from build123d import *

# Parameters (mm, degrees)
SKETCH_1_R               = 59
EXTRUDE_1_DEPTH          = 40
FILLET_1_R               = 10
SKETCH_2_R               = 5
EXTRUDE_2_DEPTH          = 5
SKETCH_3_R               = 1.75
EXTRUDE_3_DEPTH          = 5
CUT_EXTRUDE_1_DEPTH      = 93.531075925
PATTERN_CIRCULAR_1_COUNT = 6


with BuildPart() as part:
    # 草图1 → 凸台-拉伸1 (new body)
    with BuildSketch(Plane.XY):
        Circle(SKETCH_1_R)
    extrude(amount=EXTRUDE_1_DEPTH)

    # 圆角1
    fillet_1_edges = [part.edges().sort_by_distance(p)[0] for p in [
        (-59, 0, 0),
        (-59, 0, 40),
    ]]
    fillet(fillet_1_edges, radius=FILLET_1_R)

    # 草图2 → 凸台-拉伸2 (add)
    with BuildSketch(Plane.XY.offset(40)):
        Circle(SKETCH_2_R)
    extrude(amount=EXTRUDE_2_DEPTH)

    # 草图3 → 凸台-拉伸3 (add)
    with BuildSketch(Plane.XY.offset(45)):
        Circle(SKETCH_3_R)
    extrude(amount=EXTRUDE_3_DEPTH)

    # 草图4 → 切除-拉伸1 (cut, through all)
    with BuildSketch(Plane.XY.offset(40)):
        with BuildLine():
            Line((-9.6, 32.2), (-2.88, 9.16))
            ThreePointArc((-2.88, 9.16), (0, 7), (2.88, 9.16))
            Line((2.88, 9.16), (9.6, 32.2))
            ThreePointArc((9.6, 32.2), (0, 45), (-9.6, 32.2))
        make_face()
    cut_extrude_1 = extrude(amount=-CUT_EXTRUDE_1_DEPTH, mode=Mode.SUBTRACT)

    # 阵列(圆周)1: 切除-拉伸1 ×6 about axis
    pattern_circular_1_axis = Axis((0, 0, 0), (0, 0, 1))
    for i in range(1, PATTERN_CIRCULAR_1_COUNT):
        add(cut_extrude_1.rotate(pattern_circular_1_axis, i * 360 / PATTERN_CIRCULAR_1_COUNT), mode=Mode.SUBTRACT)


solid = part.part
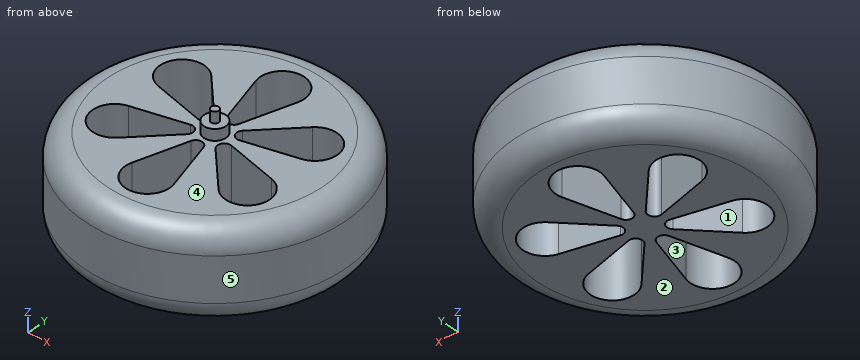
Source: CAD feature listing. Evaluate the final solid. Frame: model axes, mm. Face numbers are marked on the shaded views. A direction names the side the tool comes from. Round coordinates to 2 decimals unless told otherwise and drop trailing zeros. Loops run counter-clockwise (first coordinate to the right, second up) from the corner with the lowest first, then second, coordinate; pieces in that order, holes last. Notation, with made-up numbers: (25.25, -25) - (50.25, -25) arc R18 cw to (50.25, 8) - close; hole circle Ø9 at (-4.5, -36.5). An arc over 180 degrees is marked (long way). Write item = value, one per line. Start each with the question number.
Item 1: First-contact query: pin 1 Ø18 at (x, y) = (0, -35) entering from -Z; pin 2 Ø12 at (x, y) = (42.5, 38.5) entering from -Z; pin 3 Ø6 at (x, y) = (36, 1) entering from +Z; pin 4 Ø2 at (x, z) = (-28.5, 37) entering from -Y. Flat tips, straight axial feed; report the tip coordinate or a pass-through.
Item 2: Mould query, pull axis Y, two halves, no side actions, for the marked faces 3, 4 and 5. Classes: released by +Y, released by -Y, zero draft, split by the parting line, or undercut.
Item 3: Section query B-B on y = 0. Output: boundary loops of the cut face in (x, z), plus the area to 3 significant figures.
Item 4: Reachability of the marked faces 1 and 2 from +Z, -Z, +X, -X, +Y, -Y: full face, straight path, thin tool, end or side. Return the list, or none.
Item 5: Material intervals for line 1 (Y direction, x = 0, z = 29.5); line 2 (Y direction, x = 20, z = 9); line 3 (X direction, y = -19, z = 5), sorted ascending.
Item 6: Section query D-D on x = -12. Count the separate pieces of the cut face and the enclosed holes in it, plus the area to 3 significant figures.
Item 7: Section query C-C on z = 41.5. Output: boundary loops of the cut face in (x, y), plus the area to 3 significant figures.
Item 8: Section query A-A on z = 16. Output: boundary loops of the cut face in (x, y), plus the area to 3 significant figures.
Results list:
q1.pin_1 = through
q1.pin_2 = 0.28
q1.pin_3 = 40
q1.pin_4 = -49.53
q2.face_3 = undercut
q2.face_4 = zero draft
q2.face_5 = split by the parting line
q3.outline = (-59, 10) arc R10 ccw to (-49, 0) - (49, 0) arc R10 ccw to (59, 10) - (59, 30) arc R10 ccw to (49, 40) - (5, 40) - (5, 45) - (1.75, 45) - (1.75, 50) - (-1.75, 50) - (-1.75, 45) - (-5, 45) - (-5, 40) - (-49, 40) arc R10 ccw to (-59, 30) - close
q3.area = 4,700 mm²
q4.face_1 = +Z, -Z
q4.face_2 = -Z, +X, -X, +Y, -Y
q5.line_1 = -59 to -45, -7 to 7, 45 to 59
q5.line_2 = -55.45 to -21.19, -4.68 to 4.68, 21.19 to 55.45
q5.line_3 = -54.44 to -40.2, -17.91 to -5.75, 5.75 to 17.91, 40.2 to 54.44
q6.separate_pieces = 3
q6.enclosed_holes = 0
q6.area = 3,730 mm²
q7.outline = circle Ø10 at (0, 0)
q7.area = 78.5 mm²
q8.outline = circle Ø118 at (0, 0); hole (-32.69, -7.79) arc R10 ccw (long way) to (-23.09, -24.41) - (-6.49, -7.07) arc R3 ccw to (-9.37, -2.09) - close; hole (-32.69, 7.79) - (-9.37, 2.09) arc R3 ccw to (-6.49, 7.07) - (-23.09, 24.41) arc R10 ccw (long way) to start; hole (-9.6, -32.2) arc R10 ccw (long way) to (9.6, -32.2) - (2.88, -9.16) arc R3 ccw to (-2.88, -9.16) - close; hole (-9.6, 32.2) - (-2.88, 9.16) arc R3 ccw to (2.88, 9.16) - (9.6, 32.2) arc R10 ccw (long way) to start; hole (6.49, -7.07) - (23.09, -24.41) arc R10 ccw (long way) to (32.69, -7.79) - (9.37, -2.09) arc R3 ccw to start; hole (6.49, 7.07) arc R3 ccw to (9.37, 2.09) - (32.69, 7.79) arc R10 ccw (long way) to (23.09, 24.41) - close
q8.area = 7,880 mm²
